Geometry: see drawing. Coordinates: mm, zero at the bounding-box minimum. Coordinates: 2 decimals unless noted, no trailing zeros. Loops run counter-clockwise (first coordinate to the right, second up) from the corner with the lowest first, then second, coordinate; pieces in that order, holes last. Notation, with made-up numbers: (45, -8) -> (61, -8) arc R11 ccw to (61, 4) -> close; hole circle Ø4 at (65, 36). An arc over 180 degrees is marked (long way). Answer as a JSON object with one key per item and string values.
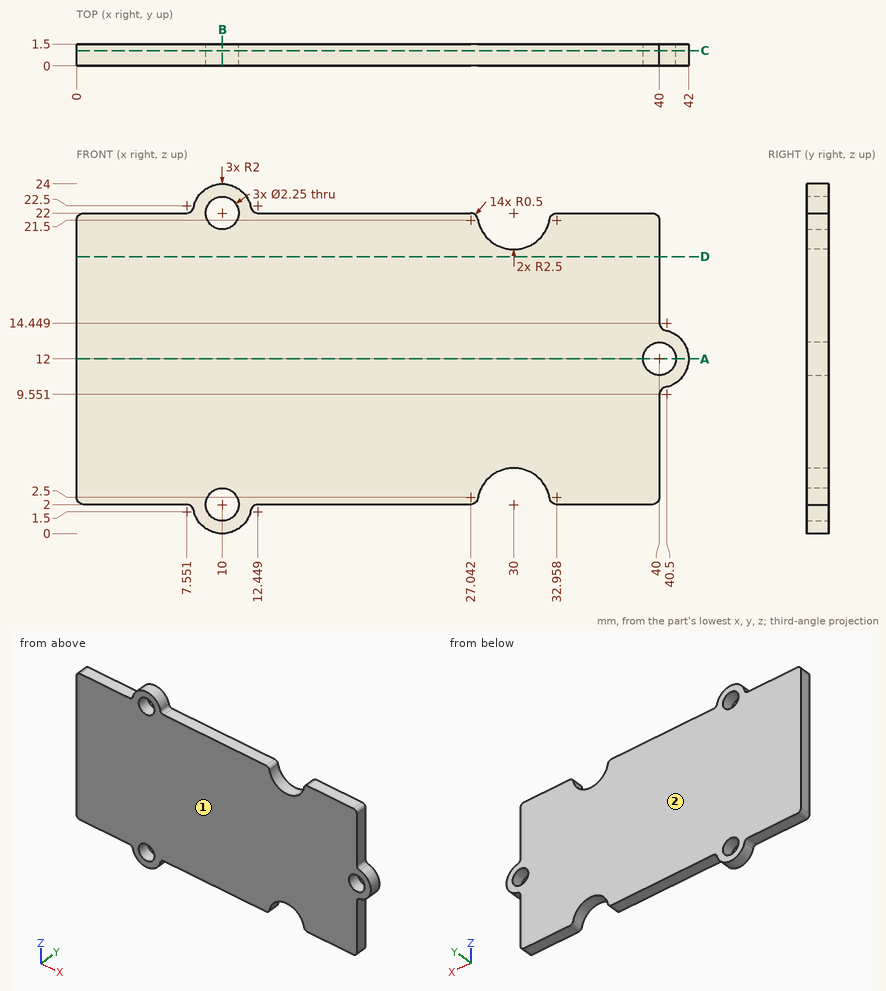
1. Section query D-D (z = 19). Return loops of the section in (x, y).
Reply:
{"outline": "(0, 0) -> (40, 0) -> (40, 1.5) -> (0, 1.5) -> close"}
2. Section query B-B (x = 10). Return loops of the section in (y, z) (1 decimal).
Reply:
{"outline": "(0, 0) -> (1.5, 0) -> (1.5, 0.9) -> (0, 0.9) -> close; (0, 3.1) -> (1.5, 3.1) -> (1.5, 20.9) -> (0, 20.9) -> close; (0, 23.1) -> (1.5, 23.1) -> (1.5, 24) -> (0, 24) -> close"}
3. Mould query, pull axis Y, two halves, no side actions, for the marked faces 1 and 2. Classes: pulls with the +Y half, pulls with the -Y half, needs draft (parallel to the pull), parting line crosses it, or undercut.
Reply:
{"face 1": "pulls with the -Y half", "face 2": "pulls with the +Y half"}
4. Pin query (flat end, axial travel): P1, Ø0.8, axis at y = 1, z = 4.5, coming from the +X side. Return the tip coordinate at first contact, or that it passes through.
Reply:
{"P1": "stops at x = 40"}
5. Section query C-C (y = 1.05). Count the separate pieces of the cut face and the enclosed holes in it, plus the area to 3 significant figures.
Reply:
{"separate pieces": "1", "enclosed holes": "3", "area": "787 mm2"}
6. Line query: line 1 along X through (y, z) = (0.95, 2.5); line 2 along X through (y, z) = (0.5, 12) (1 decimal); line 3 along Z through (x, y) = (9, 0.7) (1 decimal). Output: solid intervals per line, ascending.
Reply:
{"line 1": "x = 0 to 8.99, 11.01 to 27.55, 32.45 to 40", "line 2": "x = 0 to 38.9, 41.1 to 42", "line 3": "z = 0.3 to 1.5, 2.5 to 21.5, 22.5 to 23.7"}
7. Section query A-A (z = 12). Return loops of the section in (x, y) (1 decimal).
Reply:
{"outline": "(0, 0) -> (38.9, 0) -> (38.9, 1.5) -> (0, 1.5) -> close; (41.1, 0) -> (42, 0) -> (42, 1.5) -> (41.1, 1.5) -> close"}
